Could you check a few things on this model? Use its own coordinates, in mm. Coordinates: 2 decimals unless noted, no trailing zeros. Answer as a JSON object with one key per item and string values. Group by question number.
1) Will these pins go through, and if not, where does the flat tip stop? pin 1 Ø1.9 at (x, y) = (-17.942, 24.8) entering from -Z; pin 2 Ø4.5 at (x, y) = (17.5, -9.75) entering from +Z; pin 3 Ø1.4 at (x, y) = (-28.61, 17.942) entering from -Z.
2) If we section it at A-A (x = 10): State how many separate pieces and enclosed holes the cut face has, plus the area to 3 significant figures.
3) Please list where these lines run through material, in increasing order: line 1 along Y through (x, z) = (24.8, 3.5) (3 decimals); line 2 along X through (y, z) = (0, 1.25).
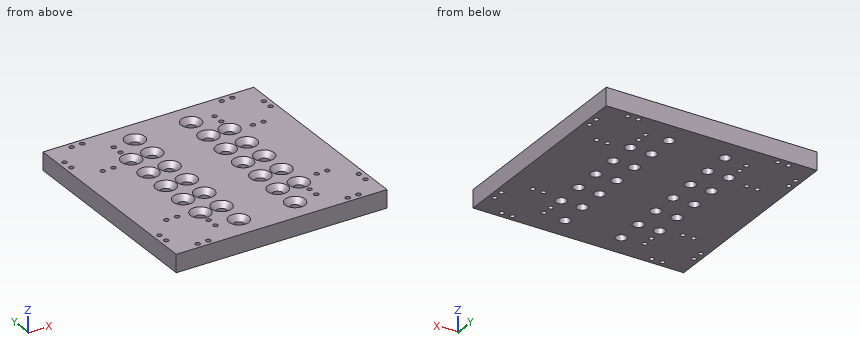
Autodesk Inventor part; units mm, degrees
ref_plane "YZ Plane" through (0, 0, 0) normal (1, 0, 0) x (0, 1, 0)
ref_plane "XZ Plane" through (0, 0, 0) normal (0, 1, 0) x (-1, 0, 0)
ref_plane "XY Plane" through (0, 0, 0) normal (0, 0, 1) x (1, 0, 0)
sketch "Sketch1" plane through (0, 0, 0) normal (0, 0, 1) x (1, 0, 0)
  line L0 (-37.5, -37.5) -> (37.5, -37.5)
  line L1 (37.5, -37.5) -> (37.5, 37.5)
  line L2 (37.5, 37.5) -> (-37.5, 37.5)
  line L3 (-37.5, 37.5) -> (-37.5, -37.5)
  line L4 (-37.5, -37.5) -> (37.5, 37.5) construction
  line L5 (37.5, -37.5) -> (-37.5, 37.5) construction
  point P0 (0, 0)
  dimension "d0" = 75
  dimension "d1" = 75
extrude "Extrusion1" add sketch "Sketch1" along normal blind 6.35
sketch "Sketch2" plane through (0, 0, 6.35) normal (0, 0, 1) x (1, 0, 0)
  line L0 (-15.91, 15.91) -> (-37.5, 15.91) construction
  line L1 (-37.5, 15.91) -> (-37.5, 37.5) construction
  line L2 (-37.5, 37.5) -> (-15.91, 37.5) construction
  line L3 (-15.91, 37.5) -> (-15.91, 15.91) construction
  line L4 (-15.91, 15.91) -> (-37.5, 37.5) construction
  line L5 (-37.5, 15.91) -> (-15.91, 37.5) construction
  line L6 (-15.91, -15.91) -> (-15.91, -37.5) construction
  line L7 (-15.91, -37.5) -> (-37.5, -37.5) construction
  line L8 (-37.5, -37.5) -> (-37.5, -15.91) construction
  line L9 (-37.5, -15.91) -> (-15.91, -15.91) construction
  line L10 (-15.91, -15.91) -> (-37.5, -37.5) construction
  line L11 (-15.91, -37.5) -> (-37.5, -15.91) construction
  line L12 (15.91, -15.91) -> (37.5, -15.91) construction
  line L13 (37.5, -15.91) -> (37.5, -37.5) construction
  line L14 (37.5, -37.5) -> (15.91, -37.5) construction
  line L15 (15.91, -37.5) -> (15.91, -15.91) construction
  line L16 (15.91, -15.91) -> (37.5, -37.5) construction
  line L17 (37.5, -15.91) -> (15.91, -37.5) construction
  line L18 (15.91, 15.91) -> (15.91, 37.5) construction
  line L19 (15.91, 37.5) -> (37.5, 37.5) construction
  line L20 (37.5, 37.5) -> (37.5, 15.91) construction
  line L21 (37.5, 15.91) -> (15.91, 15.91) construction
  line L22 (15.91, 15.91) -> (37.5, 37.5) construction
  line L23 (15.91, 37.5) -> (37.5, 15.91) construction
  line L24 (37.5, 37.5) -> (-37.5, 37.5)
  line L25 (-37.5, 37.5) -> (-37.5, -37.5)
  point P0 (0, 0)
  point P1 (-26.705, 26.705)
  point P2 (-24.8, 35.468)
  point P3 (-35.468, 24.8)
  point P4 (-35.468, 28.61)
  point P5 (-24.8, 17.942)
  point P6 (-28.61, 17.942)
  point P7 (-17.942, 28.61)
  point P8 (-17.942, 24.8)
  point P9 (-28.61, 35.468)
  point P10 (-26.705, -26.705)
  point P11 (-35.468, -28.61)
  point P12 (-24.8, -17.942)
  point P13 (-28.61, -17.942)
  point P14 (-17.942, -28.61)
  point P15 (-17.942, -24.8)
  point P16 (-28.61, -35.468)
  point P17 (-24.8, -35.468)
  point P18 (-35.468, -24.8)
  point P19 (26.705, -26.705)
  point P20 (28.61, -35.468)
  point P21 (17.942, -24.8)
  point P22 (17.942, -28.61)
  point P23 (28.61, -17.942)
  point P24 (24.8, -17.942)
  point P25 (35.468, -28.61)
  point P26 (35.468, -24.8)
  point P27 (24.8, -35.468)
  point P28 (26.705, 26.705)
  point P29 (35.468, 28.61)
  point P30 (24.8, 17.942)
  point P31 (28.61, 17.942)
  point P32 (17.942, 28.61)
  point P33 (17.942, 24.8)
  point P34 (28.61, 35.468)
  point P35 (24.8, 35.468)
  point P36 (35.468, 24.8)
  dimension "d4" = 21.59
  dimension "d5" = 21.59
  dimension "d6" = 2.032
  dimension "d7" = 12.7
  dimension "d10" = 360
  dimension "d15" = 360
hole "Hole1" at (-24.8, 35.468, 6.35) at (-35.468, 24.8, 6.35) at (-35.468, 28.61, 6.35) at (-24.8, 17.942, 6.35) at (-28.61, 17.942, 6.35) at (-17.942, 28.61, 6.35) at (-17.942, 24.8, 6.35) at (-28.61, 35.468, 6.35) at (-35.468, -28.61, 6.35) at (-24.8, -17.942, 6.35) at (-28.61, -17.942, 6.35) at (-17.942, -28.61, 6.35) at (-17.942, -24.8, 6.35) at (-28.61, -35.468, 6.35) at (-24.8, -35.468, 6.35) at (-35.468, -24.8, 6.35) at (28.61, -35.468, 6.35) at (17.942, -24.8, 6.35) at (17.942, -28.61, 6.35) at (28.61, -17.942, 6.35) at (24.8, -17.942, 6.35) at (35.468, -28.61, 6.35) at (35.468, -24.8, 6.35) at (24.8, -35.468, 6.35) at (35.468, 28.61, 6.35) at (24.8, 17.942, 6.35) at (28.61, 17.942, 6.35) at (17.942, 28.61, 6.35) at (17.942, 24.8, 6.35) at (28.61, 35.468, 6.35) at (24.8, 35.468, 6.35) at (35.468, 24.8, 6.35) direction (0, 0, -1) diameter 1.694 depth 6.637 tip angle 118
sketch "Sketch3" plane through (0, 0, 6.35) normal (0, 0, 1) x (1, 0, 0)
  line L0 (-37.5, 37.5) -> (-37.5, -37.5) construction
  line L1 (37.5, -37.5) -> (37.5, 37.5) construction
  line L2 (37.5, 37.5) -> (-37.5, 37.5) construction
  line L3 (-37.5, 37.5) -> (-37.5, -37.5) construction
  line L4 (-17.5, -19.5) -> (17.5, -19.5) construction
  line L5 (37.5, 37.5) -> (-37.5, 37.5) construction
  line L6 (-37.5, -37.5) -> (37.5, -37.5) construction
  circle A0 centre (-17.942, 24.8) radius 0.847
  circle A1 centre (-17.942, -24.8) radius 0.847
  point P0 (-17.5, -9.75)
  point P1 (17.5, -9.75)
  point P2 (-17.5, 0)
  point P3 (17.5, 0)
  point P4 (-17.5, 9.75)
  point P5 (17.5, 9.75)
  point P6 (-17.5, 19.5)
  point P7 (17.5, 19.5)
  dimension "d67" = 35
  dimension "d97" = 18
  dimension "d114" = 9.75
hole "Hole7" at (-17.5, -19.5, 6.35) at (17.5, -19.5, 6.35) at (-17.5, -9.75, 6.35) at (17.5, -9.75, 6.35) at (-17.5, 0, 6.35) at (17.5, 0, 6.35) at (-17.5, 9.75, 6.35) at (17.5, 9.75, 6.35) at (-17.5, 19.5, 6.35) at (17.5, 19.5, 6.35) direction (0, 0, -1) diameter 3.797 depth 10.979 tip angle 118 countersink diameter 7.087 countersink angle 82
sketch "Sketch4" plane through (0, 0, 6.35) normal (0, 0, 1) x (1, 0, 0)
  circle A0 centre (-17.5, -19.5) radius 1.8985 construction
  circle A1 centre (17.5, -19.5) radius 1.8985 construction
  circle A2 centre (17.5, -19.5) radius 1.8985 construction
  line L0 (-17.5, -19.5) -> (17.5, -19.5) construction
  line L1 (0, 0) -> (0, -37.5) construction
  line L2 (-37.5, -37.5) -> (37.5, -37.5) construction
  point P0 (-10, -19.5)
  point P1 (10, -19.5)
  point P2 (-10, -9.75)
  point P3 (10, -9.75)
  point P4 (-10, 0)
  point P5 (10, 0)
  point P6 (-10, 9.75)
  point P7 (10, 9.75)
  point P8 (-10, 19.5)
  point P9 (10, 19.5)
  point P10 (-10, 29.25)
  point P11 (10, 29.25)
  point P12 (-10, -29.25)
  point P13 (10, -29.25)
  point P14 (-10, -19.5)
  point P15 (10, -19.5)
  point P16 (-10, -9.75)
  point P17 (10, -9.75)
  point P18 (-10, 0)
  point P19 (10, 0)
  point P20 (-10, 9.75)
  point P21 (10, 9.75)
  point P22 (-10, 19.5)
  point P23 (10, 19.5)
  dimension "d126" = 10
  dimension "d129" = 9.75
  dimension "d132" = 9.75
hole "Hole8" at (-10, -19.5, 6.35) at (10, -19.5, 6.35) at (-10, -9.75, 6.35) at (10, -9.75, 6.35) at (-10, 0, 6.35) at (10, 0, 6.35) at (-10, 9.75, 6.35) at (10, 9.75, 6.35) at (-10, 19.5, 6.35) at (10, 19.5, 6.35) at (-10, 29.25, 6.35) at (10, 29.25, 6.35) at (-10, -29.25, 6.35) at (10, -29.25, 6.35) direction (0, 0, -1) diameter 3.797 depth 10.979 tip angle 118 countersink diameter 7.087 countersink angle 82
properties part number "6dof_plate"
Here are the results:
{
 "1": {"pin 1": "stops at z = 0", "pin 2": "stops at z = 4.86", "pin 3": "passes through"},
 "2": {"separate pieces": "8", "enclosed holes": "0", "area": "286 mm²"},
 "3": {"line 1": "y = -37.5 to -36.315, -34.621 to -18.789, -17.095 to 17.095, 18.789 to 34.621, 36.315 to 37.5", "line 2": "x = -37.5 to -19.4, -15.6 to -11.9, -8.1 to 8.1, 11.9 to 15.6, 19.4 to 37.5"}
}
